from build123d import *

# Parameters (mm, degrees)
CUT_EXTRUDE1_DEPTH      = 67.516915142
CUT_EXTRUDE1_DEPTH_BACK = 67.516915142
SKETCH2_R               = 2.75
SKETCH2_R_2             = 2.5
SKETCH3_W               = 7
SKETCH3_H               = 4
CUT_EXTRUDE2_DEPTH      = 5
BOSS_EXTRUDE1_START     = -20
SKETCH5_R               = 2.75
BOSS_EXTRUDE1_DEPTH     = 20


with BuildPart() as part:
    # Sketch1 → Revolve1 (revolve)
    with BuildSketch(Plane.XY, mode=Mode.PRIVATE) as revolve1_sk:
        Polygon((-28, 10), (-46.5, 10), (-46.5, 0), (-13, 0), (-13, 7), (-28, 7), align=None)
    revolve(revolve1_sk.sketch.rotate(Axis((0, -1.751877994, 0), (0, 1, 0)), 270), axis=Axis((0, -1.751877994, 0), (0, 1, 0)))

    # Sketch2 → Cut-Extrude1 (cut, two sides: drawn at the far end of the back side and taken through both)
    with BuildSketch(Plane(origin=(0, 10, 0), x_dir=(1, 0, 0), z_dir=(0, 1, 0)).offset(-CUT_EXTRUDE1_DEPTH_BACK)):
        with Locations(Location((0, 41, 0), (0, 0, 270))):
            Circle(SKETCH2_R)
        with Locations(Location((15.690020727, 37.879060833, 0), (0, 0, 270))):
            Circle(SKETCH2_R_2)
        with Locations(Location((28.991378029, 28.991378029, 0), (0, 0, 270))):
            Circle(SKETCH2_R)
        with Locations(Location((37.879060833, 15.690020727, 0), (0, 0, 270))):
            Circle(SKETCH2_R_2)
        with Locations(Location((41, 0, 0), (0, 0, 270))):
            Circle(SKETCH2_R)
        with Locations(Location((37.879060833, -15.690020727, 0), (0, 0, 270))):
            Circle(SKETCH2_R_2)
        with Locations(Location((28.991378029, -28.991378029, 0), (0, 0, 270))):
            Circle(SKETCH2_R)
        with Locations(Location((15.690020727, -37.879060833, 0), (0, 0, 270))):
            Circle(SKETCH2_R_2)
        with Locations(Location((0, -41, 0), (0, 0, 270))):
            Circle(SKETCH2_R)
        with Locations(Location((-15.690020727, -37.879060833, 0), (0, 0, 270))):
            Circle(SKETCH2_R_2)
        with Locations(Location((-28.991378029, -28.991378029, 0), (0, 0, 270))):
            Circle(SKETCH2_R)
        with Locations(Location((-37.879060833, -15.690020727, 0), (0, 0, 270))):
            Circle(SKETCH2_R_2)
        with Locations(Location((-41, 0, 0), (0, 0, 270))):
            Circle(SKETCH2_R)
        with Locations(Location((-37.879060833, 15.690020727, 0), (0, 0, 270))):
            Circle(SKETCH2_R_2)
        with Locations(Location((-28.991378029, 28.991378029, 0), (0, 0, 270))):
            Circle(SKETCH2_R)
        with Locations(Location((-15.690020727, 37.879060833, 0), (0, 0, 270))):
            Circle(SKETCH2_R_2)
    extrude(amount=CUT_EXTRUDE1_DEPTH + CUT_EXTRUDE1_DEPTH_BACK, mode=Mode.SUBTRACT)

    # Sketch3 → Cut-Revolve1 (revolve, cut)
    with BuildSketch(Plane.XY, mode=Mode.PRIVATE) as cut_revolve1_sk:
        with Locations((25, 2)):
            Rectangle(SKETCH3_W, SKETCH3_H)
    revolve(cut_revolve1_sk.sketch.rotate(Axis((0, -19.065406541, 0), (0, 1, 0)), 90), axis=Axis((0, -19.065406541, 0), (0, 1, 0)), mode=Mode.SUBTRACT)

    # Sketch4 → Cut-Extrude2 (cut)
    with BuildSketch(Plane.XZ):
        Polygon((-19.690020727, 40.18846191), (-19.690020727, 35.569659756), (-15.690020727, 33.260258679), (-11.690020727, 35.569659756), (-11.690020727, 40.18846191), (-15.690020727, 42.497862986), align=None)
        Polygon((18.956007051, 41.145047157), (14.494586764, 42.34048112), (11.22860044, 39.074494796), (12.424034403, 34.613074509), (16.88545469, 33.417640546), (20.151441014, 36.68362687), align=None)
        Polygon((42.497862986, 15.690020727), (40.18846191, 19.690020727), (35.569659756, 19.690020727), (33.260258679, 15.690020727), (35.569659756, 11.690020727), (40.18846191, 11.690020727), align=None)
        Polygon((41.145047157, -18.956007051), (42.34048112, -14.494586764), (39.074494796, -11.22860044), (34.613074509, -12.424034403), (33.417640546, -16.88545469), (36.68362687, -20.151441014), align=None)
        Polygon((15.690020727, -42.497862986), (19.690020727, -40.18846191), (19.690020727, -35.569659756), (15.690020727, -33.260258679), (11.690020727, -35.569659756), (11.690020727, -40.18846191), align=None)
        Polygon((-18.956007051, -41.145047157), (-14.494586764, -42.34048112), (-11.22860044, -39.074494796), (-12.424034403, -34.613074509), (-16.88545469, -33.417640546), (-20.151441014, -36.68362687), align=None)
        Polygon((-42.497862986, -15.690020727), (-40.18846191, -19.690020727), (-35.569659756, -19.690020727), (-33.260258679, -15.690020727), (-35.569659756, -11.690020727), (-40.18846191, -11.690020727), align=None)
        Polygon((-41.145047157, 18.956007051), (-42.34048112, 14.494586764), (-39.074494796, 11.22860044), (-34.613074509, 12.424034403), (-33.417640546, 16.88545469), (-36.68362687, 20.151441014), align=None)
    extrude(amount=-CUT_EXTRUDE2_DEPTH, mode=Mode.SUBTRACT)

    # Sketch5 → Boss-Extrude1 (add)
    with BuildSketch(Plane.XZ.offset(BOSS_EXTRUDE1_START)):
        with Locations(Location((0, 41, 0), (0, 0, 270))):
            Circle(SKETCH5_R)
        with Locations(Location((28.991378029, 28.991378029, 0), (0, 0, 270))):
            Circle(SKETCH5_R)
        with Locations(Location((41, 0, 0), (0, 0, 270))):
            Circle(SKETCH5_R)
        with Locations(Location((28.991378029, -28.991378029, 0), (0, 0, 270))):
            Circle(SKETCH5_R)
        with Locations(Location((0, -41, 0), (0, 0, 270))):
            Circle(SKETCH5_R)
        with Locations(Location((-28.991378029, -28.991378029, 0), (0, 0, 270))):
            Circle(SKETCH5_R)
        with Locations(Location((-41, 0, 0), (0, 0, 270))):
            Circle(SKETCH5_R)
        with Locations(Location((-28.991378029, 28.991378029, 0), (0, 0, 270))):
            Circle(SKETCH5_R)
    extrude(amount=BOSS_EXTRUDE1_DEPTH)


solid = part.part
Geometry check sheet. Reference: the model listing, model coordinates, mm. A direction names the side the tool comes from. Round coordinates to 2 decimals unless told otherwise and drop trailing zeros. Write each loop counter-clockwise with the first axis right and the second up, starting at its lowest first coordinate (ties: lowest second). Pieces come first, ordered by that corner, then holes.
Item 1: Go/stop test with flat-tipped pins: pin 1 Ø6 at (x, z) = (15.69, 37.88) entering from -Y; pin 2 Ø12 at (y, z) = (14.5, -16.5) entering from -X; pin 3 Ø6 at (x, z) = (37.88, -15.69) entering from +Y. Record where each tip stops, or that it passes through.
Determined:
pin 1: stops at y = 5
pin 2: stops at x = -44.78
pin 3: stops at y = 10
Item 2: Section check A-A (z = 0). Record the boundary of the cut face in (x, y), plus the area to 3 significant figures.
Determined:
outline: (-46.5, 0) - (-28.5, 0) - (-28.5, 4) - (-21.5, 4) - (-21.5, 0) - (-13, 0) - (-13, 7) - (-28, 7) - (-28, 10) - (-38.25, 10) - (-38.25, 20) - (-43.75, 20) - (-43.75, 10) - (-46.5, 10) - close; (13, 0) - (21.5, 0) - (21.5, 4) - (28.5, 4) - (28.5, 0) - (46.5, 0) - (46.5, 10) - (43.75, 10) - (43.75, 20) - (38.25, 20) - (38.25, 10) - (28, 10) - (28, 7) - (13, 7) - close
area: 634 mm2
Item 3: Material ranges on line 1 along X through (y, z) = (1.45, 0); line 2 along X through (y, z) = (4.5, 15); line 3 along Y through (x, z) = (28, -10.5), recorded low to high.
Determined:
line 1: x = -46.5 to -28.5, -21.5 to -13, 13 to 21.5, 28.5 to 46.5
line 2: x = -44.01 to -42.21, -33.92 to 33.66, 42.1 to 44.01
line 3: y = 0 to 10
Item 4: Section check C-C (y = 13.75). Record the boundary of the cut face in (x, z).
Determined:
outline: circle Ø5.5 at (-41, 0); circle Ø5.5 at (-28.99, -28.99); circle Ø5.5 at (-28.99, 28.99); circle Ø5.5 at (0, -41); circle Ø5.5 at (0, 41); circle Ø5.5 at (28.99, -28.99); circle Ø5.5 at (28.99, 28.99); circle Ø5.5 at (41, 0)
Item 5: Section check B-B (x = 0). Record the boundary of the cut face in (y, z), plus the area to 3 significant figures.
Determined:
outline: (0, -46.5) - (10, -46.5) - (10, -43.75) - (20, -43.75) - (20, -38.25) - (10, -38.25) - (10, -28) - (7, -28) - (7, -13) - (0, -13) - (0, -21.5) - (4, -21.5) - (4, -28.5) - (0, -28.5) - close; (0, 13) - (7, 13) - (7, 28) - (10, 28) - (10, 38.25) - (20, 38.25) - (20, 43.75) - (10, 43.75) - (10, 46.5) - (0, 46.5) - (0, 28.5) - (4, 28.5) - (4, 21.5) - (0, 21.5) - close
area: 634 mm2
Item 6: Access from +Z, -Z, +X, -X, +Y, -Y to the whole of each face (thin tool, end or side, straight path). Record for faces 1 (the face through (7.91, 3.549, 10.316)), 2 (the face through (-14.624, 2.465, -34.024)), 3 (the face through (-28.165, 15.07, 26.368)).
Determined:
face 1: +Y, -Y
face 2: -Y
face 3: +Y
Item 7: Section check D-D (x = 23.5). Record the boundary of the cut face in (y, z), plus the area to 3 significant figures.
Determined:
outline: (0, -40.12) - (10, -40.12) - (10, -15.22) - (7, -15.22) - (7, 15.22) - (10, 15.22) - (10, 40.12) - (0, 40.12) - (0, 16.12) - (4, 16.12) - (4, -16.12) - (0, -16.12) - close
area: 582 mm2
Item 8: Mould release check, pull along X, two halves, no side actions. Record for faces 4 (the face through (-29, 20, -29)), 5 (the face through (-40, 5, 14)): +X half, -X half, draft (parallel to the pull), parting line (faces both ways), or undercut.
Determined:
face 4: draft
face 5: undercut
